from build123d import *

# Parameters (mm, degrees)
SKETCH1_R           = 8.25
BOSS_EXTRUDE1_DEPTH = 9.1
SKETCH2_R           = 3.5
BOSS_EXTRUDE2_DEPTH = 6.5
SKETCH3_R           = 3.175
BOSS_EXTRUDE3_DEPTH = 8.5
BOSS_EXTRUDE4_START = -0.5
BOSS_EXTRUDE4_DEPTH = 0.5
SKETCH5_W           = 4
SKETCH5_H           = 0.5
BOSS_EXTRUDE5_DEPTH = 10.2
SKETCH6_W           = 1
SKETCH6_H           = 0.5
BOSS_EXTRUDE6_DEPTH = 5
CUT_EXTRUDE1_REACH  = 26.054
SKETCH7_W           = 1.25
SKETCH7_H           = 5.244370441
SKETCH7_W_2         = 1


with BuildPart() as part:
    # Sketch1 → Boss-Extrude1 (new body)
    with BuildSketch(Plane(origin=(0, 0, 0), x_dir=(1, 0, 0), z_dir=(0, 1, 0))):
        with Locations(Location((0, 0, 0), (0, 0, 270))):
            Circle(SKETCH1_R)
    extrude(amount=BOSS_EXTRUDE1_DEPTH)

    # Sketch2 → Boss-Extrude2 (add)
    with BuildSketch(Plane(origin=(0, 9.1, 0), x_dir=(1, 0, 0), z_dir=(0, 1, 0))):
        with Locations(Location((0, 0, 0), (0, 0, 90))):
            Circle(SKETCH2_R)
    extrude(amount=BOSS_EXTRUDE2_DEPTH)

    # Sketch3 → Boss-Extrude3 (add)
    with BuildSketch(Plane(origin=(0, 15.6, 0), x_dir=(1, 0, 0), z_dir=(0, 1, 0))):
        with Locations(Location((0, 0, 0), (0, 0, 270))):
            Circle(SKETCH3_R)
    extrude(amount=BOSS_EXTRUDE3_DEPTH)

    # Sketch4 → Boss-Extrude4 (add)
    with BuildSketch(Plane(origin=(0, 9.1, 0), x_dir=(1, 0, 0), z_dir=(0, 1, 0)).offset(BOSS_EXTRUDE4_START)):
        with BuildLine():
            Line((-8.25, 0), (-8.25, -16.25))
            Line((-8.25, -16.25), (8.25, -16.25))
            Line((8.25, -16.25), (8.25, 0))
            ThreePointArc((8.25, 0), (0, -8.25), (-8.25, 0))
        make_face()
    extrude(amount=BOSS_EXTRUDE4_DEPTH)

    # Sketch5 → Boss-Extrude5 (add)
    with BuildSketch(Plane.XZ.offset(-8.6)):
        with Locations((0, 16)):
            Rectangle(SKETCH5_W, SKETCH5_H)
        with Locations((-5, 16)):
            Rectangle(SKETCH5_W, SKETCH5_H)
        with Locations((5, 16)):
            Rectangle(SKETCH5_W, SKETCH5_H)
    extrude(amount=BOSS_EXTRUDE5_DEPTH)

    # Sketch6 → Boss-Extrude6 (add)
    with BuildSketch(Plane.XZ.offset(1.6)):
        with Locations((5, 16)):
            Rectangle(SKETCH6_W, SKETCH6_H)
        with Locations((0, 16)):
            Rectangle(SKETCH6_W, SKETCH6_H)
        with Locations((-5, 16)):
            Rectangle(SKETCH6_W, SKETCH6_H)
    extrude(amount=BOSS_EXTRUDE6_DEPTH)

    # Sketch7 → Cut-Extrude1 (cut, up to next)
    with BuildSketch(Plane(origin=(0, 9.1, 0), x_dir=(1, 0, 0), z_dir=(0, 1, 0)), mode=Mode.PRIVATE) as cut_extrude1_sk1:
        with Locations((-7.625, -13.627814779)):
            Rectangle(SKETCH7_W, SKETCH7_H)
    cut_extrude1_tool1 = extrude(cut_extrude1_sk1.sketch, amount=-CUT_EXTRUDE1_REACH, mode=Mode.PRIVATE) & part.part
    # Sketch7 → Cut-Extrude1 (cut, up to next)
    with BuildSketch(Plane(origin=(0, 9.1, 0), x_dir=(1, 0, 0), z_dir=(0, 1, 0)), mode=Mode.PRIVATE) as cut_extrude1_sk2:
        with Locations((7.625, -13.627814779)):
            Rectangle(SKETCH7_W, SKETCH7_H)
    cut_extrude1_tool2 = extrude(cut_extrude1_sk2.sketch, amount=-CUT_EXTRUDE1_REACH, mode=Mode.PRIVATE) & part.part
    # Sketch7 → Cut-Extrude1 (cut, up to next)
    with BuildSketch(Plane(origin=(0, 9.1, 0), x_dir=(1, 0, 0), z_dir=(0, 1, 0)), mode=Mode.PRIVATE) as cut_extrude1_sk3:
        with Locations((2.5, -13.627814779)):
            Rectangle(SKETCH7_W_2, SKETCH7_H)
    cut_extrude1_tool3 = extrude(cut_extrude1_sk3.sketch, amount=-CUT_EXTRUDE1_REACH, mode=Mode.PRIVATE) & part.part
    # Sketch7 → Cut-Extrude1 (cut, up to next)
    with BuildSketch(Plane(origin=(0, 9.1, 0), x_dir=(1, 0, 0), z_dir=(0, 1, 0)), mode=Mode.PRIVATE) as cut_extrude1_sk4:
        with Locations((-2.5, -13.627814779)):
            Rectangle(SKETCH7_W_2, SKETCH7_H)
    cut_extrude1_tool4 = extrude(cut_extrude1_sk4.sketch, amount=-CUT_EXTRUDE1_REACH, mode=Mode.PRIVATE) & part.part
    add(cut_extrude1_tool1.solids().sort_by_distance((-7.625, 9.1, 13.627815))[0], mode=Mode.SUBTRACT)
    add(cut_extrude1_tool2.solids().sort_by_distance((7.625, 9.1, 13.627815))[0], mode=Mode.SUBTRACT)
    add(cut_extrude1_tool3.solids().sort_by_distance((2.5, 9.1, 13.627815))[0], mode=Mode.SUBTRACT)
    add(cut_extrude1_tool4.solids().sort_by_distance((-2.5, 9.1, 13.627815))[0], mode=Mode.SUBTRACT)


solid = part.part
Input: part model. Units: mm. Frame: model coordinates. A direction names the side the tool comes from. Coordinates: 2 decimals unless noted, no trailing zeros. Loops run counter-clockwise (first coordinate to the right, second up) from the corner with the lowest first, then second, coordinate; pieces in that order, holes last. Notation, with made-up numbers: (24.25, -40) -> (65.25, -40) arc R24 cw to (65.25, -18) -> close; hole circle Ø4 at (50.5, 38.25). An arc over 180 degrees is marked (long way). One line per item, written item: value.
(1) Cut plane C-C (y = -2). Output: boundary loops of the cut face in (x, z).
Answer below:
outline: (-5.5, 15.75) -> (-4.5, 15.75) -> (-4.5, 16.25) -> (-5.5, 16.25) -> close; (-0.5, 15.75) -> (0.5, 15.75) -> (0.5, 16.25) -> (-0.5, 16.25) -> close; (4.5, 15.75) -> (5.5, 15.75) -> (5.5, 16.25) -> (4.5, 16.25) -> close
(2) Cut plane D-D (x = 0). Output: boundary loops of the cut face in (y, z) (3 decimals).
Answer below:
outline: (-6.6, 15.75) -> (8.6, 15.75) -> (8.6, 8.25) -> (0, 8.25) -> (0, -8.25) -> (9.1, -8.25) -> (9.1, -3.5) -> (15.6, -3.5) -> (15.6, -3.175) -> (24.1, -3.175) -> (24.1, 3.175) -> (15.6, 3.175) -> (15.6, 3.5) -> (9.1, 3.5) -> (9.1, 16.25) -> (-6.6, 16.25) -> close
(3) Cut plane A-A (y = 6.5). Output: boundary loops of the cut face in (x, z), then the cut area to 3 significant figures.
Answer below:
outline: circle Ø16.5 at (0, 0); (-7, 15.75) -> (-3, 15.75) -> (-3, 16.25) -> (-7, 16.25) -> close; (-2, 15.75) -> (2, 15.75) -> (2, 16.25) -> (-2, 16.25) -> close; (3, 15.75) -> (7, 15.75) -> (7, 16.25) -> (3, 16.25) -> close
area: 220 mm2
(4) Ray query, line 1 along Y through (x, z) = (-3.75, 10); line 2 along Y through (x, z) = (6.5, -2.75); line 3 along Z through (x, y) = (3.5, 7.5). Return the intervals inside material, ascending.
Answer below:
line 1: y = 8.6 to 9.1
line 2: y = 0 to 9.1
line 3: z = -7.47 to 7.47, 15.75 to 16.25
(5) Draft query along Z for faces 5 (the face through (2, 5, 16)), 6 (the face through (0, 3, 16.25)), 7 (the face through (-5, 3, 15.75)). Return one class per face: pulls with the +Z half, pulls with the -Z half, needs draft (parallel to the pull), parting line crosses it, or undercut.
Answer below:
face 5: needs draft
face 6: pulls with the +Z half
face 7: undercut
(6) Cut plane B-B (z = 14.75). Output: boundary loops of the cut face in (x, y), then the cut area to 3 significant figures.
Answer below:
outline: (-7, 8.6) -> (-3, 8.6) -> (-3, 9.1) -> (-7, 9.1) -> close; (-2, 8.6) -> (2, 8.6) -> (2, 9.1) -> (-2, 9.1) -> close; (3, 8.6) -> (7, 8.6) -> (7, 9.1) -> (3, 9.1) -> close
area: 6.00 mm2
(7) Set-up query: faces 1 (the face through (2.48, 4.49, 7.87)), 2 (the face through (-7, 5, 16)), 3 (the face through (0, 3, 15.75)), 4 (the face through (-2, 5, 16)). Return all of +Z, -Z, +X, -X, +Y, -Y with unobstructed straight access to the full face (end or side cutting, diameter ignored); none if empty.
Answer below:
face 1: -Y
face 2: +Z, -X, +Y, -Y
face 3: +X, -X, -Y
face 4: +Z, +Y, -Y
(8) Pin query (flat end, axial travel): pin 1 Ø8 at (x, z) = (-2, 8.5) entering from -Y; pin 2 Ø6 at (x, z) = (-2.5, 10) entering from +Y; pin 3 Ø0.6 at (x, y) = (2.5, 9) entering from +Z; pin 4 Ø4 at (y, z) = (4, 13) entering from -X. Return the tip coordinate at first contact, or that it passes through.
Answer below:
pin 1: stops at y = 0
pin 2: stops at y = 9.1
pin 3: stops at z = 11.01
pin 4: passes through
